from build123d import *

# Parameters (mm, degrees)
BOSS_EXTRUDE1_DEPTH = 4
CUT_EXTRUDE1_DEPTH  = 4


with BuildPart() as part:
    # Sketch1 → Boss-Extrude1 (new body)
    with BuildSketch(Plane(origin=(0, 0, 0), x_dir=(1, 0, 0), z_dir=(0, 1, 0))):
        Polygon((-115, 60), (115, 60), (115, 20), (111, 20), (111, -20), (115, -20), (115, -60), (-115, -60), (-115, -20), (-111, -20), (-111, 20), (-115, 20), align=None)
    extrude(amount=BOSS_EXTRUDE1_DEPTH)

    # Sketch2 → Cut-Extrude1 (cut)
    with BuildSketch(Plane.XZ):
        with BuildLine():
            Line((-87.5, -35), (-87.5, 35))
            ThreePointArc((-87.5, 35), (-85, 37.5), (-82.5, 35))
            Line((-82.5, 35), (-82.5, -35))
            ThreePointArc((-82.5, -35), (-85, -37.5), (-87.5, -35))
        make_face()
        with BuildLine():
            Line((-72.5, -35), (-72.5, 35))
            ThreePointArc((-72.5, 35), (-70, 37.5), (-67.5, 35))
            Line((-67.5, 35), (-67.5, -35))
            ThreePointArc((-67.5, -35), (-70, -37.5), (-72.5, -35))
        make_face()
        with BuildLine():
            Line((-57.5, -35), (-57.5, 35))
            ThreePointArc((-57.5, 35), (-55, 37.5), (-52.5, 35))
            Line((-52.5, 35), (-52.5, -35))
            ThreePointArc((-52.5, -35), (-55, -37.5), (-57.5, -35))
        make_face()
        with BuildLine():
            Line((-42.5, -35), (-42.5, 35))
            ThreePointArc((-42.5, 35), (-40, 37.5), (-37.5, 35))
            Line((-37.5, 35), (-37.5, -35))
            ThreePointArc((-37.5, -35), (-40, -37.5), (-42.5, -35))
        make_face()
        with BuildLine():
            Line((-27.5, -35), (-27.5, 35))
            ThreePointArc((-27.5, 35), (-25, 37.5), (-22.5, 35))
            Line((-22.5, 35), (-22.5, -35))
            ThreePointArc((-22.5, -35), (-25, -37.5), (-27.5, -35))
        make_face()
        with BuildLine():
            Line((87.5, -35), (87.5, 35))
            ThreePointArc((87.5, 35), (85, 37.5), (82.5, 35))
            Line((82.5, 35), (82.5, -35))
            ThreePointArc((82.5, -35), (85, -37.5), (87.5, -35))
        make_face()
        with BuildLine():
            Line((72.5, -35), (72.5, 35))
            ThreePointArc((72.5, 35), (70, 37.5), (67.5, 35))
            Line((67.5, 35), (67.5, -35))
            ThreePointArc((67.5, -35), (70, -37.5), (72.5, -35))
        make_face()
        with BuildLine():
            Line((57.5, -35), (57.5, 35))
            ThreePointArc((57.5, 35), (55, 37.5), (52.5, 35))
            Line((52.5, 35), (52.5, -35))
            ThreePointArc((52.5, -35), (55, -37.5), (57.5, -35))
        make_face()
        with BuildLine():
            Line((42.5, -35), (42.5, 35))
            ThreePointArc((42.5, 35), (40, 37.5), (37.5, 35))
            Line((37.5, 35), (37.5, -35))
            ThreePointArc((37.5, -35), (40, -37.5), (42.5, -35))
        make_face()
        with BuildLine():
            Line((27.5, -35), (27.5, 35))
            ThreePointArc((27.5, 35), (25, 37.5), (22.5, 35))
            Line((22.5, 35), (22.5, -35))
            ThreePointArc((22.5, -35), (25, -37.5), (27.5, -35))
        make_face()
    extrude(amount=-CUT_EXTRUDE1_DEPTH, mode=Mode.SUBTRACT)


solid = part.part
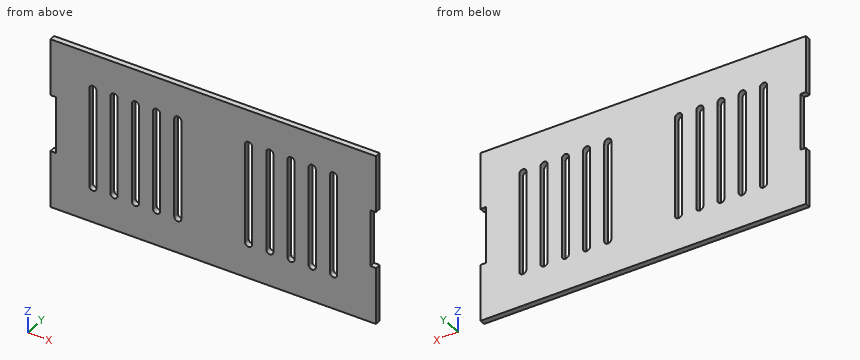
Build history of the part. All positions in model axes, mm. Coordinates: 2 decimals unless noted, no trailing zeros. Write each loop counter-clockwise with the first axis right and the second up, starting at its lowest first coordinate (ties: lowest second). Pieces come first, ordered by that corner, then holes.
(1) Cut at B-B on y = 1.7. State how many separate pieces and enclosed holes the cut face has, and give its area (3 significant figures).
(2) Cut at A-A on x = -40. List the corners of the cut face in (y, z).
(3) Pin check, flat tips, straight feed: pin 1 Ø1.2 at (y, z) = (1.5, -1.5) entering from -X; pin 2 Ø2 at (y, z) = (3, 15.5) entering from +X. Stop position of each tip, or through.
(4) Drill centre lines: line 1 (Z direction, x = -25.5, y = 1.2); line 2 (Z direction, x = 71, y = 0.5). Where is each one in solid material? Low to high.
Working result:
1. separate pieces: 1
1. enclosed holes: 10
1. area: 23,600 mm2
2. outline: (0, -60) - (4, -60) - (4, -37.5) - (0, -37.5) - close; (0, 37.5) - (4, 37.5) - (4, 60) - (0, 60) - close
3. pin 1: stops at x = -111
3. pin 2: stops at x = 111
4. line 1: z = -60 to -37.45, 37.45 to 60
4. line 2: z = -60 to -37.29, 37.29 to 60
